Can you work these out from the model? Positions are in its coordinate system, mm. A direction names the side the tool comes from. Give positions to 0.01 mm unless a question says otherwise; leave off trailing zeros. Order: outer loops, then holes, each group sorted by start corner. A loop starts at its lowest first (then second) coordinate and runs counter-clockwise, first axis right, second up.
Item 1: I want a section at B-B, the plane y = -52.5. Write out the boundary of the cut face in (x, z), then the cut area to 3 significant figures.
Item 2: I want a section at C-C, the plane z = 0.55. Write out the boundary of the cut face in (x, y).
Item 3: Which directions (+Z, -Z, +X, -X, +Y, -Y) give clear straight access to the entire face, cutting with the end or side of a thin tool? Please do faces 1 (the flat face through (-62, -59, 1)), 2 (the flat face through (-15, -59, 3)), 3 (the flat face through (1, -29, 1)).
Item 4: If I drill on line 1 along X through (y, z) = (-49, 2.5); line 2 along Y through (x, z) = (-99.5, 2.9); line 3 along Y through (x, z) = (-23, 1.05), over which ranges is the centre line in solid material (lowest first)?
Item 5: I want a section at A-A, the plane x = -40.5. Write out the boundary of the cut face in (y, z).
Item 6: I'm going to push flat-ended pins straight in: pin 1 Ø1.6 at (x, z) = (-60.5, 1.5) entering from -Y; pin 2 Ø2 at (x, y) = (-61, 2) entering from +Z. Where does each tip first touch, or does it pass through?
Item 7: If we mould it in two halves opening along Y, with no side actions, what happens to faces 4 (the flat face through (-62.4, 3, 0.8)), 5 (the flat face through (-124, -29, 1)), 6 (the flat face through (-108, -59, 3))? For each: +Y half, -Y half, draft (parallel to the pull), parting line (faces both ways), or undercut.
Item 8: I want a section at D-D, the plane y = -28. Write out the boundary of the cut face in (x, z), then the cut area to 3 significant figures.
```python
from build123d import *

# Parameters (mm, degrees)
F0_W     = 129
F0_H     = 64
F0_W_2   = 123
F0_H_2   = 58
F0_W_3   = 121
F0_H_3   = 56
F1_DEPTH = 2
F2_W     = 129
F2_H     = 64
F3_DEPTH = 1
F4_W     = 15
F4_H     = 36.0279009569
F4_H_2   = 3
F4_H_3   = 6.1532862581
F4_W_2   = 4
F4_H_4   = 15
F4_W_3   = 3.5279009569
F4_W_4   = 37.6532862581
F5_DEPTH = 2


with BuildPart() as f1:
    # F0 (on Top) → F1 (new body)
    with BuildSketch(Plane.XY):
        with Locations((-61.5, -29)):
            Rectangle(F0_W, F0_H)
        with Locations((-61.5, -29)):
            Rectangle(F0_W_2, F0_H_2, mode=Mode.SUBTRACT)
        with Locations((-61.5, -29)):
            Rectangle(F0_W_2, F0_H_2)
        with Locations((-61.5, -29)):
            Rectangle(F0_W_3, F0_H_3, mode=Mode.SUBTRACT)
    extrude(amount=F1_DEPTH)

    # F2 (on face) → F3 (join)
    with BuildSketch(Plane.XY.offset(2)):
        with Locations((-61.5, -29)):
            Rectangle(F2_W, F2_H)
        Polygon((-122, 0), (-1, 0), (-1, -1), (-1, -57), (-1, -58), (-122, -58), (-122, -57), (-122, -1), align=None, mode=Mode.SUBTRACT)
    extrude(amount=F3_DEPTH)

    # F4 (on face) → F5 (cut)
    with BuildSketch(Plane.XY.offset(3)):
        with Locations((-61.5, 21.0139504785)):
            Rectangle(F4_W, F4_H)
        with Locations((-61.5, 1.5)):
            Rectangle(F4_W, F4_H_2)
        with Locations((-61.5, -3.0766431291)):
            Rectangle(F4_W, F4_H_3)
        with Locations((1, -29)):
            Rectangle(F4_W_2, F4_H_4)
        with Locations((4.7639504785, -29)):
            Rectangle(F4_W_3, F4_H_4)
        with Locations((-19.8266431291, -29)):
            Rectangle(F4_W_4, F4_H_4)
        with Locations((-61.5, -59.5)):
            Rectangle(F4_W, F4_H_2)
        with Locations((-61.5, -54.9233568709)):
            Rectangle(F4_W, F4_H_3)
        with Locations((-61.5, -79.0139504785)):
            Rectangle(F4_W, F4_H)
        with Locations((-103.1733568709, -29)):
            Rectangle(F4_W_4, F4_H_4)
        with Locations((-124, -29)):
            Rectangle(F4_W_2, F4_H_4)
        with Locations((-127.7639504785, -29)):
            Rectangle(F4_W_3, F4_H_4)
    extrude(amount=-F5_DEPTH, mode=Mode.SUBTRACT)


solid = f1.part
```
Results list:
1. outline: (-126, 0) - (-122, 0) - (-122, 3) - (-126, 3) - close; (-1, 0) - (3, 0) - (3, 3) - (-1, 3) - close
1. area: 24.0 mm2
2. outline: (-126, -61) - (3, -61) - (3, 3) - (-126, 3) - close; hole (-122, -57) - (-1, -57) - (-1, -1) - (-122, -1) - close
3. face 1: +Z, +Y, -Y
3. face 2: +Z, +X, -X, +Y, -Y
3. face 3: +Z, +X, -X
4. line 1: x = -126 to -122, -1 to 3
4. line 2: y = -61 to -58, 0 to 3
4. line 3: y = -61 to -57, -1 to 3
5. outline: (-61, 0) - (-57, 0) - (-57, 2) - (-58, 2) - (-58, 3) - (-61, 3) - close; (-1, 0) - (3, 0) - (3, 3) - (0, 3) - (0, 2) - (-1, 2) - close
6. pin 1: stops at y = -61
6. pin 2: stops at z = 1
7. face 4: +Y half
7. face 5: undercut
7. face 6: draft
8. outline: (-126, 0) - (-122, 0) - (-122, 1) - (-126, 1) - close; (-1, 0) - (3, 0) - (3, 1) - (-1, 1) - close
8. area: 8.00 mm2
